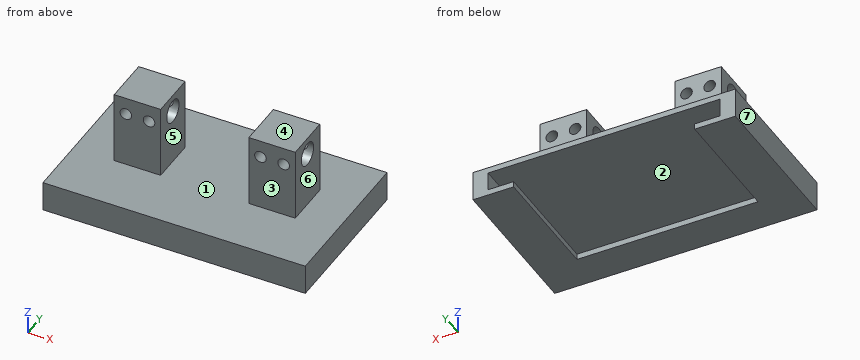
from build123d import *

# Parameters (mm, degrees)
SKETCH3_W               = 226
SKETCH3_H               = 133.5
BOSS_EXTRUDE1_DEPTH     = 26
SKETCH4_W               = 200
SKETCH4_H               = 16
CUT_EXTRUDE2_DEPTH      = 64.5
CUT_EXTRUDE2_DEPTH_BACK = 60
SKETCH6_W               = 40
SKETCH6_H               = 40
BOSS_EXTRUDE5_DEPTH     = 63
SKETCH7_R               = 10
CUT_EXTRUDE3_DEPTH      = 260
SKETCH13_R              = 5
CUT_EXTRUDE6_DEPTH      = 91
SKETCH10_W              = 156
SKETCH10_H              = 103.5
CUT_EXTRUDE5_DEPTH      = 5


with BuildPart() as part:
    # Sketch3 → Boss-Extrude1 (new body)
    with BuildSketch(Plane.XY):
        with Locations((0, -3.25)):
            Rectangle(SKETCH3_W, SKETCH3_H)
    extrude(amount=BOSS_EXTRUDE1_DEPTH)

    # Sketch4 → Cut-Extrude2 (cut, two sides)
    with BuildSketch(Plane(origin=(0, 0, 0), x_dir=(1, 0, 0), z_dir=(0, 1, 0))) as cut_extrude2_sk:
        with Locations((0, -13)):
            Rectangle(SKETCH4_W, SKETCH4_H)
    extrude(amount=CUT_EXTRUDE2_DEPTH, mode=Mode.SUBTRACT)
    extrude(cut_extrude2_sk.sketch, amount=-CUT_EXTRUDE2_DEPTH_BACK, mode=Mode.SUBTRACT)

    # Sketch6 → Boss-Extrude5 (add)
    with BuildSketch(Plane.XY.offset(26)):
        with Locations((-58, 0)):
            Rectangle(SKETCH6_W, SKETCH6_H)
        with Locations((58, 0)):
            Rectangle(SKETCH6_W, SKETCH6_H)
    extrude(amount=BOSS_EXTRUDE5_DEPTH)

    # Sketch7 → Cut-Extrude3 (cut)
    with BuildSketch(Plane(origin=(113, 0, 0), x_dir=(0, 0, -1), z_dir=(1, 0, 0))):
        with Locations((-74, 0)):
            Circle(SKETCH7_R)
    extrude(amount=-CUT_EXTRUDE3_DEPTH, mode=Mode.SUBTRACT)

    # Sketch13 → Cut-Extrude6 (cut, through all)
    with BuildSketch(Plane(origin=(0, 20, 0), x_dir=(1, 0, 0), z_dir=(0, 1, 0))):
        with Locations((-68, -74)):
            Circle(SKETCH13_R)
        with Locations((-48, -74)):
            Circle(SKETCH13_R)
        with Locations((48, -74)):
            Circle(SKETCH13_R)
        with Locations((68, -74)):
            Circle(SKETCH13_R)
    extrude(amount=-CUT_EXTRUDE6_DEPTH, mode=Mode.SUBTRACT)

    # Sketch10 → Cut-Extrude5 (cut)
    with BuildSketch(Plane(origin=(0, 0, 0), x_dir=(-1, 0, 0), z_dir=(0, 0, -1))):
        with Locations((0, 11.75)):
            Rectangle(SKETCH10_W, SKETCH10_H)
    extrude(amount=-CUT_EXTRUDE5_DEPTH, mode=Mode.SUBTRACT)


solid = part.part
Here's how the part is built. I have some questions about the finished solid (model axes, mm). Face numbers are marked on the shaded views. A direction names the side the tool comes from. Give positions to 0.01 mm unless a question says otherwise; leave off trailing zeros. Write each loop counter-clockwise with the first axis right and the second up, starting at its lowest first coordinate (ties: lowest second). Pieces come first, ordered by that corner, then holes. Notation, with made-up numbers: (53.5, -24.75) -> (66.5, -24.75) arc R18 cw to (66.5, -6.75) -> close; hole circle Ø11 at (-9.5, 41.25). An arc over 180 degrees is marked (long way). Use one line per item in the form item = value. Start each with the question number.
1. Will these pins go through, and if not, where does the flat tip stop? pin 1 Ø12 at (y, z) = (-9.5, 50) entering from +X; pin 2 Ø20 at (x, z) = (-67.5, 70) entering from +Y; pin 3 Ø1.5 at (x, y) = (-36.5, 32) entering from +Z.
2. On a 3-axis mill with a long thin cutter (end or side, diameter ignored), from which of +Z, -Z, +X, -X, +Y, -Y can I reach the whole of each face in a straight line? I mean the marked faces 1, 2, 3 and 4. Say none if no direction works.
3. Imagine slicing it at A-A on x = -68. List the corners of the cut face in (y, z) for me.
4. Imagine slicing it at C-C on y = 0. List the corners of the cut face in (x, z) for me, plus the area to 3 significant figures.
5. If I drill on L1, parallel to X at y = 13, z = 74; L2, parallel to Z at x = -95, y = -28; L3, parallel to X at y = 32.5, z = 17, over which ranges is the centre line in solid material (lowest first)?
6. Imagine slicing it at B-B on z = 49. List the corners of the cut face in (x, y) for me.
7. Imagine slicing it at D-D on y = -43.5. List the corners of the cut face in (x, z) for me, plus the area to 3 significant figures.
8. Thinking about a two-plate mould opening in X: for the marked faces 5, 6 and 7, which applies, +X half, -X half, draft (parallel to the pull), parting line (faces both ways), or undercut?
Entries:
q1.pin_1 = 78
q1.pin_2 = 20
q1.pin_3 = 26
q2.face_1 = +Z
q2.face_2 = +Y
q2.face_3 = +Z, +X, -X, -Y
q2.face_4 = +Z, +X, -X, +Y, -Y
q3.outline = (-70, 0) -> (-40, 0) -> (-40, 5) -> (-60, 5) -> (-60, 21) -> (63.5, 21) -> (63.5, 26) -> (20, 26) -> (20, 69) -> (8.66, 69) arc R10 cw to (-8.66, 69) -> (-20, 69) -> (-20, 26) -> (-70, 26) -> close; (-20, 79) -> (-8.66, 79) arc R10 cw to (8.66, 79) -> (20, 79) -> (20, 89) -> (-20, 89) -> close
q4.outline = (-113, 0) -> (-78, 0) -> (-78, 5) -> (-100, 5) -> (-100, 21) -> (100, 21) -> (100, 5) -> (78, 5) -> (78, 0) -> (113, 0) -> (113, 26) -> (78, 26) -> (78, 64) -> (38, 64) -> (38, 26) -> (-38, 26) -> (-38, 64) -> (-78, 64) -> (-78, 26) -> (-113, 26) -> close; (-78, 84) -> (-38, 84) -> (-38, 89) -> (-78, 89) -> close; (38, 84) -> (78, 84) -> (78, 89) -> (38, 89) -> close
q4.area = 5,340 mm²
q5.L1 = -78 to -73, -63 to -53, -43 to -38, 38 to 43, 53 to 63, 73 to 78
q5.L2 = 0 to 5, 21 to 26
q5.L3 = -113 to -100, 100 to 113
q6.outline = (-78, -20) -> (-38, -20) -> (-38, 20) -> (-78, 20) -> close; (38, -20) -> (78, -20) -> (78, 20) -> (38, 20) -> close
q7.outline = (-113, 0) -> (113, 0) -> (113, 26) -> (-113, 26) -> close; hole (-100, 5) -> (100, 5) -> (100, 21) -> (-100, 21) -> close
q7.area = 2,680 mm²
q8.face_5 = undercut
q8.face_6 = +X half
q8.face_7 = -X half
